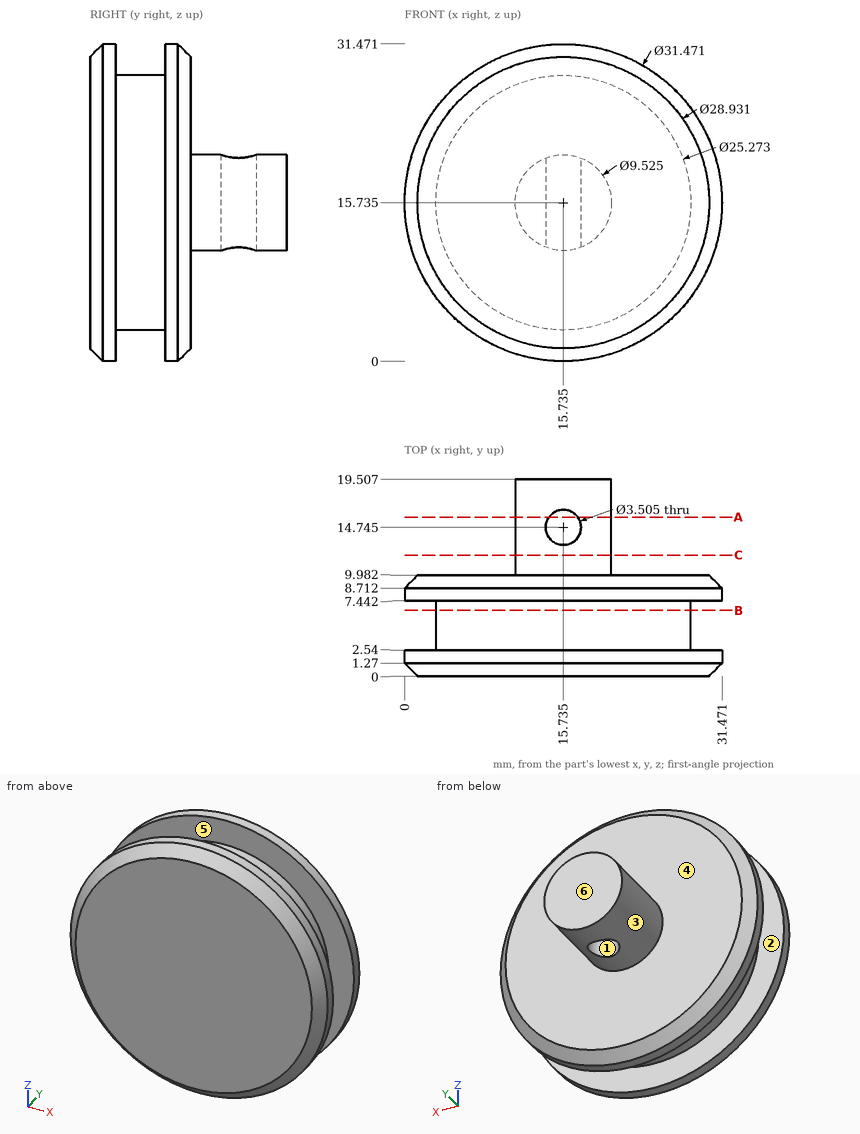
Geometry check sheet. Reference: drawing and pictorial views, mm from the part's lowest x, y, z. A direction names the side the tool comes from. Give positions to 0.01 mm unless a question says otherwise; leave off trailing zeros. Order: outer loops, then holes, each group sorted by start corner. A loop starts at its lowest first (then second) coordinate and runs counter-clockwise, first axis right, second up. Notation, with made-up numbers: (-10, -35.5) - (7, -35.5) arc R23 cw to (7, -27.5) - close; hole circle Ø8 at (71, 39.25). An arc over 180 degrees is marked (long way). Use one line per item in the form item = value.
1) Sectioned sample at C-C (y = 12). Record the boundary of the cut face in (x, z) (1 decimal).
Working result:
outline = circle Ø9.5 at (15.7, 15.7)
2) Depth check by flat-ended pin: pin 1 Ø3 at (x, y) = (14, 14) entering from +Z; pin 2 Ø4 at (y, z) = (8, 5) entering from +X; pin 3 Ø5 at (x, z) = (7.5, 16) entering from +Y; pin 4 Ø3 at (y, z) = (13.5, 23.5) entering from +X. Enter the tip coordinate at first touch or a pass-through.
Working result:
pin_1 = 20.47
pin_2 = 28.82
pin_3 = 9.98
pin_4 = through
3) Draft check along X on the marked faces 1, 2 and 3. Enter one of: released by +X, released by -X, zero draft, split by the parting line, or undercut.
Working result:
face_1 = undercut
face_2 = zero draft
face_3 = split by the parting line
4) Sectioned sample at B-B (y = 6.5). Record the boundary of the cut face in (x, z) (1 decimal), and give its area (3 significant figures).
Working result:
outline = circle Ø25.3 at (15.7, 15.7)
area = 502 mm^2
5) Access from +Z, -Z, +X, -X, +Y, -Y to the whole of each face (thin tool, end or side, straight path). Record for the marked faces 4, 5 and 6.
Working result:
face_4 = +Y
face_5 = none
face_6 = +Z, -Z, +X, -X, +Y
6) Sectioned sample at A-A (y = 15.75). Record the boundary of the cut face in (x, z) (1 decimal).
Working result:
outline = (14.3, 11.2) - (14.3, 20.3) arc R4.8 ccw to start; (17.2, 11.2) arc R4.8 ccw to (17.2, 20.3) - close
7) Material ranges on probe 1 along Y at (x, z) = (25, 5); probe 2 along Y at (x, z) = (6, 14); probe 3 along X at (y, z) = (13.75, 17) (1 decimal), recorded low to high. Write a range as from..to.
Working result:
probe_1 = 0..2.54, 7.44..9.98
probe_2 = 0..9.98
probe_3 = 11.1..14.3, 17.2..20.3
